CAD build for the part. Positions are in the model's coordinates, mm. A direction names the side the tool comes from. Give positions to 0.01 mm unless a question says otherwise; leave off trailing zeros. Loops run counter-clockwise (first coordinate to the right, second up) from the corner with the lowest first, then second, coordinate; pieces in that order, holes last. Notation, with made-up numbers: M 34.5,45 L 61.5,45 A16 ccw 61.5,60 Z; hole C 79.25,-23.75 d5. An arc over 180 degrees is marked long. Answer as CSV lines item,"result".
```python
from build123d import *

# Parameters (mm, degrees)
ESTRUSIONE_ESTRUSIONE1_DEPTH = 16
SCHIZZO2_R                   = 3.25
TAGLIO_ESTRUSIONE1_DEPTH     = 4
TAGLIO_ESTRUSIONE2_DEPTH     = 4
SCHIZZO4_R                   = 3.25
TAGLIO_ESTRUSIONE3_DEPTH     = 3
TAGLIO_ESTRUSIONE5_DEPTH     = 3


with BuildPart() as part:
    # Schizzo1 → Estrusione-Estrusione1 (new body)
    with BuildSketch(Plane.XY):
        Polygon((0, 20), (0, 0), (25, 0), (25, -5), (-5, -5), (-5, 20), align=None)
    extrude(amount=ESTRUSIONE_ESTRUSIONE1_DEPTH)

    # Schizzo2 → Taglio-Estrusione1 (cut)
    with BuildSketch(Plane(origin=(0, 0, 0), x_dir=(0, 0, -1), z_dir=(1, 0, 0))):
        with Locations(Location((-8, 12.5, 0), (0, 0, 90))):
            Circle(SCHIZZO2_R)
    extrude(amount=-TAGLIO_ESTRUSIONE1_DEPTH, mode=Mode.SUBTRACT)

    # Schizzo3 → Taglio-Estrusione2 (cut)
    with BuildSketch(Plane(origin=(0, 0, 0), x_dir=(1, 0, 0), z_dir=(0, 1, 0))):
        with BuildLine():
            Line((17.25, -5.25), (17.25, -10.5))
            ThreePointArc((17.25, -10.5), (19, -12.25), (20.75, -10.5))
            Line((20.75, -10.5), (20.75, -5.25))
            ThreePointArc((20.75, -5.25), (19, -3.5), (17.25, -5.25))
        make_face()
        with BuildLine():
            Line((7.75, -5.25), (7.75, -10.5))
            ThreePointArc((7.75, -10.5), (9.5, -12.25), (11.25, -10.5))
            Line((11.25, -10.5), (11.25, -5.25))
            ThreePointArc((11.25, -5.25), (9.5, -3.5), (7.75, -5.25))
        make_face()
    extrude(amount=-TAGLIO_ESTRUSIONE2_DEPTH, mode=Mode.SUBTRACT)

    # Schizzo4 → Taglio-Estrusione3 (cut)
    with BuildSketch(Plane(origin=(-4, 0, 0), x_dir=(0, 0, -1), z_dir=(1, 0, 0))):
        with Locations(Location((-8, 12.5, 0), (0, 0, 90))):
            Circle(SCHIZZO4_R)
    extrude(amount=-TAGLIO_ESTRUSIONE3_DEPTH, mode=Mode.SUBTRACT)

    # Schizzo5 → Taglio-Estrusione5 (cut)
    with BuildSketch(Plane(origin=(0, -4, 0), x_dir=(1, 0, 0), z_dir=(0, 1, 0))):
        with BuildLine():
            Line((11.268981919, -5.25), (11.268981919, -10.5))
            ThreePointArc((11.268981919, -10.5), (9.5, -12.268981919), (7.731018081, -10.5))
            Line((7.731018081, -10.5), (7.731018081, -5.25))
            ThreePointArc((7.731018081, -5.25), (9.5, -3.481018081), (11.268981919, -5.25))
        make_face()
        with BuildLine():
            Line((20.769481266, -5.25), (20.769481266, -10.5))
            ThreePointArc((20.769481266, -10.5), (19.000499347, -12.268981919), (17.231517428, -10.5))
            Line((17.231517428, -10.5), (17.231517428, -5.25))
            ThreePointArc((17.231517428, -5.25), (19.000499347, -3.481018081), (20.769481266, -5.25))
        make_face()
    extrude(amount=-TAGLIO_ESTRUSIONE5_DEPTH, mode=Mode.SUBTRACT)


solid = part.part
```
Q1. Cut at D-D (z = 14.25). Write the cut outline in (x, y), and give its area (3 significant figures).
Solution:
outline,"M -5,-5 L 25,-5 L 25,0 L 0,0 L 0,20 L -5,20 Z"
area,"250 mm²"
Q2. Pin check, flat tip, straight feed: P1, Ø8, axis at x = 15.5, z = 11, coming from the +Y side. Stop position of the tip, or through.
Solution:
P1,"stops at y = 0"
Q3. Wall check: line 1 (Z direction, x = -1.75, y = 12.5); line 2 (X direction, y = -3, z = 7.5); line 3 (X direction, y = 8, z = 12.5). Give the ranges that are in metal, low to high. Write a range as [from, to].
Solution:
line 1,"z = [0, 4.75], [11.25, 16]"
line 2,"x = [-5, 7.75], [11.25, 17.25], [20.75, 25]"
line 3,"x = [-5, 0]"
Q4. Which spindle directions (+Z, -Z, +X, -X, +Y, -Y) get a long thin tool onto all of the face, cutting with end or side? Do faces 1 (the flat face through (0, 8, 8)), 2 (the flat face through (20.75, -2, 8)), 3 (the flat face through (-5, 7, 8)). Say none if no direction does.
Solution:
face 1,"+Z, -Z, +X, +Y"
face 2,"+Y, -Y"
face 3,"+Z, -Z, -X, +Y, -Y"
Q5. Cut at A-A (y = 12.5). Write the cut outline in (x, z), and give its area (3 significant figures).
Solution:
outline,"M -5,0 L 0,0 L 0,4.75 L -5,4.75 Z; M -5,11.25 L 0,11.25 L 0,16 L -5,16 Z"
area,"47.5 mm²"
Q6. Mould opens along Y. For faces 4 (the flat face through (12, 0, 8)), 5 (the cylindrical face through (-2.465, 10.105, 10.197)), 6 (the cylindrical face through (18.96, -4.49, 3.48)) say: released by +Y, released by -Y, zero draft, split by the parting line, or undercut.
Solution:
face 4,"released by +Y"
face 5,"undercut"
face 6,"zero draft"
Q7. Cut at B-B (z = 8). Give the number of separate pieces and of enclosed holes in the cut face, and give its area (3 significant figures).
Solution:
separate pieces,"4"
enclosed holes,"0"
area,"182 mm²"
